Work out the finished part from the listing and answer in its coordinate system (mm). A direction names the side the tool comes from. Give positions to 0.01 mm unless a question says otherwise; leave off trailing zeros. Loops run counter-clockwise (first coordinate to the right, second up) from the corner with the lowest first, then second, coordinate; pieces in that order, holes last. Notation, with made-up numbers: (50, 80) - (57, 80) arc R21 ccw to (57, 114) - close; hole circle Ø4 at (53.25, 42.5). An arc over 180 degrees is marked (long way). One line per question, with ' | ' between items. Start each with the question number.
1. Each of these flat-tipped pins is pushed along its axis until it touches: pin 1 (15.5 mm diameter, centred on y = 6.5, z = 9.5, fed in from +X); pin 2 (1.2 mm diameter, centred on y = -26, z = -35.5, fed in from +X). Where does it stop, or does it pass through?
2. Section D-D (x = 8.5) is taken. Determine the outline of the cut face in (y, z).
3. Section C-C (y = 1) is taken. Determine the outline of the cut face in (x, z), plus the area to 3 significant figures.
4. Section B-B (z = 34.75) is taken. Determine the outline of the cut face in (x, y), plus the area to 3 significant figures.
5. For a pull along Y with two mould halves and no side action, classify faces 3 (the face through (0, 0, 1)), 4 (the face through (58, 0, 31)), 5 (the face through (55, 30.5, 1)) as released by +Y, released by -Y, zero draft, split by the parting line, or undercut.
6. Which of the six approach directions +Z, -Z, +X, -X, +Y, -Y give full straight-line access (tool end or side, diameter ignored) to faces 1 (the face through (97, 26, 35)), 2 (the face through (112, 28, 1))?
7. Section A-A (x = 104.5) is taken. Determine the outline of the cut face in (y, z), plus the area to 3 significant figures.
8. Find the intervals of material crossed by line 1 (Y direction, x = 108, z = -34.75); line 2 (Y direction, x = 105.5, z = -10.5); line 3 (Z direction, x = 78.5, y = 14), in increasing order.
from build123d import *

# Parameters (mm, degrees)
CROQUIS1_W              = 77
CROQUIS1_H              = 61
SALIENTE_EXTRUIR1_DEPTH = 112
CROQUIS3_W              = 62
CROQUIS3_H              = 52
CORTAR_EXTRUIR4_DEPTH   = 110
CROQUIS10_R             = 2
CORTAR_EXTRUIR5_DEPTH   = 15
REDONDEO1_R             = 2
REDONDEO2_R             = 2


with BuildPart() as part:
    # Croquis1 → Saliente-Extruir1 (new body)
    with BuildSketch(Plane(origin=(0, 0, 0), x_dir=(0, 0, -1), z_dir=(1, 0, 0))):
        Rectangle(CROQUIS1_W, CROQUIS1_H)
    extrude(amount=SALIENTE_EXTRUIR1_DEPTH)

    # Croquis3 → Cortar-Extruir4 (cut)
    with BuildSketch(Plane(origin=(112, 0, 0), x_dir=(0, 0, -1), z_dir=(1, 0, 0))):
        Rectangle(CROQUIS3_W, CROQUIS3_H)
    extrude(amount=-CORTAR_EXTRUIR4_DEPTH, mode=Mode.SUBTRACT)

    # Croquis10 → Cortar-Extruir5 (cut)
    with BuildSketch(Plane(origin=(112, 0, 0), x_dir=(0, 0, -1), z_dir=(1, 0, 0))):
        with Locations((-34.75, 25.5)):
            Circle(CROQUIS10_R)
        with Locations((34.75, 25.5)):
            Circle(CROQUIS10_R)
        with Locations((34.75, -25.5)):
            Circle(CROQUIS10_R)
        with Locations((-34.75, -25.5)):
            Circle(CROQUIS10_R)
    extrude(amount=-CORTAR_EXTRUIR5_DEPTH, mode=Mode.SUBTRACT)

    # Redondeo1
    redondeo1_edges = [part.edges().sort_by_distance(p)[0] for p in [
        (56, 30.5, 38.5),
    ]]
    fillet(redondeo1_edges, radius=REDONDEO1_R)

    # Redondeo2
    redondeo2_edges = [part.edges().sort_by_distance(p)[0] for p in [
        (56, -30.5, -38.5),
        (56, -30.5, 38.5),
        (56, 30.5, -38.5),
    ]]
    fillet(redondeo2_edges, radius=REDONDEO2_R)


solid = part.part
Conclusion:
1) pin 1: x = 2 | pin 2: x = 97
2) outline: (-30.5, -36.5) arc R2 ccw to (-28.5, -38.5) - (28.5, -38.5) arc R2 ccw to (30.5, -36.5) - (30.5, 36.5) arc R2 ccw to (28.5, 38.5) - (-28.5, 38.5) arc R2 ccw to (-30.5, 36.5) - close; hole (-26, -31) - (26, -31) - (26, 31) - (-26, 31) - close
3) outline: (0, -38.5) - (112, -38.5) - (112, -31) - (2, -31) - (2, 31) - (112, 31) - (112, 38.5) - (0, 38.5) - close | area: 1,800 mm²
4) outline: (0, -30.5) - (112, -30.5) - (112, -27.5) - (97, -27.5) - (97, -23.5) - (112, -23.5) - (112, 23.5) - (97, 23.5) - (97, 27.5) - (112, 27.5) - (112, 30.5) - (0, 30.5) - close | area: 6,710 mm²
5) face 3: zero draft | face 4: undercut | face 5: released by +Y
6) face 1: +X | face 2: +Z, -Z, +X, +Y, -Y
7) outline: (-30.5, -36.5) arc R2 ccw to (-28.5, -38.5) - (28.5, -38.5) arc R2 ccw to (30.5, -36.5) - (30.5, 36.5) arc R2 ccw to (28.5, 38.5) - (-28.5, 38.5) arc R2 ccw to (-30.5, 36.5) - close; hole circle Ø4 at (-25.5, -34.75); hole circle Ø4 at (-25.5, 34.75); hole (-26, -31) - (26, -31) - (26, 31) - (-26, 31) - close; hole circle Ø4 at (25.5, -34.75); hole circle Ø4 at (25.5, 34.75) | area: 1,420 mm²
8) line 1: -30.5 to -27.5, -23.5 to 23.5, 27.5 to 30.5 | line 2: -30.5 to -26, 26 to 30.5 | line 3: -38.5 to -31, 31 to 38.5
